Autodesk Inventor part; units mm, degrees
ref_plane "Work Plane1" through (-287.5, 0, 0) normal (0, -1, 0) x (1, 0, 0)
ref_plane "YZ Plane" through (0, 0, 0) normal (1, 0, 0) x (0, 1, 0)
ref_plane "XZ Plane" through (0, 0, 0) normal (0, 1, 0) x (-1, 0, 0)
sketch "Sketch1" plane through (0, 0, 0) normal (0, 0, 1) x (1, 0, 0)
  line L0 (137.5, -75) -> (-137.5, -75)
  line L1 (-137.5, -75) -> (-137.5, 75)
  line L2 (-137.5, 75) -> (137.5, 75)
  line L3 (137.5, 75) -> (137.5, -75)
  line L4 (137.5, -75) -> (-137.5, 75) construction
  line L5 (-137.5, -75) -> (137.5, 75) construction
  line L6 (187.5, 125) -> (-187.5, 125)
  line L7 (-187.5, 125) -> (-187.5, -125)
  line L8 (-187.5, -125) -> (187.5, -125)
  line L9 (187.5, -125) -> (187.5, 125)
  line L10 (-187.5, 125) -> (-287.5, 125)
  line L11 (-287.5, 125) -> (-287.5, 75)
  line L12 (-287.5, 75) -> (-187.5, 75)
  line L13 (-187.5, 75) -> (-187.5, 125)
  line L14 (-187.5, -75) -> (-287.5, -75)
  line L15 (-287.5, -75) -> (-287.5, -125)
  line L16 (-287.5, -125) -> (-187.5, -125)
  line L17 (-187.5, -125) -> (-187.5, -75)
  line L18 (0, 175) -> (0, -175) construction
  line L19 (-1719.5601, 0) -> (1799.9601, 0) construction
  line L20 (187.5, 125) -> (287.5, 125)
  line L21 (287.5, 125) -> (287.5, 75)
  line L22 (287.5, 75) -> (187.5, 75)
  line L23 (187.5, -75) -> (287.5, -75)
  line L24 (287.5, -75) -> (287.5, -125)
  line L25 (287.5, -125) -> (187.5, -125)
  line L26 (1719.5601, 0) -> (-1799.9601, 0) construction
  point P0 (0, 0)
  point P1 (237.5, -125)
  point P2 (0, -125)
  point P3 (-237.5, 125)
  point P4 (0, 125)
  point P5 (237.5, 125)
  point P6 (-237.5, -125)
  point P7 (-237.5, -75)
  point P8 (0, -75)
  point P9 (-237.5, 75)
  point P10 (0, 75)
  point P11 (-287.5, 100)
  point P12 (-287.5, -100)
  point P13 (287.5, 100)
  point P14 (287.5, -100)
  point P15 (187.5, 75)
  dimension "d0" = 50
  dimension "d1" = 150
  dimension "d2" = 275
  dimension "d3" = 100
extrude "Extrusion1" add sketch "Sketch1" along normal blind 30
ref_plane "Work Plane1" through (-287.5, 0, 0) normal (0, -1, 0) x (1, 0, 0)
sketch "Sketch2" plane through (-287.5, 0, 0) normal (0, -1, 0) x (1, 0, 0)
  line L0 (475, 30) -> (475, 0) construction
  line L1 (475, 0) -> (425, 0) construction
  line L2 (425, 0) -> (425, 30) construction
  line L3 (425, 30) -> (475, 30) construction
  line L4 (100, 0) -> (100, 30) construction
  line L5 (100, 30) -> (150, 30) construction
  line L6 (150, 30) -> (150, 0) construction
  line L7 (150, 0) -> (100, 0) construction
  line L8 (475, 30) -> (475, 0) construction
  line L9 (475, 0) -> (425, 0) construction
  line L10 (425, 0) -> (425, 30) construction
  line L11 (100, 0) -> (100, 30) construction
  line L12 (150, 30) -> (150, 0) construction
  line L13 (150, 0) -> (100, 0) construction
  line L14 (0, 0) -> (100, 0) construction
  line L15 (100, 0) -> (100, 30) construction
  line L16 (0, 30) -> (100, 30) construction
  line L17 (0, 0) -> (0, 30) construction
  line L18 (150, 0) -> (425, 0) construction
  line L19 (425, 0) -> (425, 30) construction
  line L20 (150, 30) -> (425, 30) construction
  line L21 (150, 0) -> (150, 30) construction
  line L22 (475, 0) -> (575, 0) construction
  line L23 (575, 0) -> (575, 30) construction
  line L24 (475, 30) -> (575, 30) construction
  line L25 (475, 0) -> (475, 30) construction
  line L26 (0, 0) -> (0, 30)
  line L27 (0, 0) -> (100, 30)
  line L28 (475, 30) -> (575, 0)
  line L29 (425, 30) -> (475, 30)
  line L30 (100, 30) -> (150, 30)
  line L31 (0, 0) -> (100, 0)
  line L32 (100, 30) -> (100, 0)
  line L33 (475, 30) -> (475, 0)
  line L34 (575, 0) -> (0, 0)
  line L35 (575, 0) -> (475, 0)
  line L36 (0, 30) -> (100, 30)
  line L37 (100, 30) -> (100, 0)
  line L38 (100, 0) -> (0, 0)
  line L39 (0, 0) -> (0, 30)
  line L40 (475, 30) -> (575, 30)
  line L41 (575, 30) -> (575, 0)
  line L42 (575, 0) -> (475, 0)
  line L43 (475, 0) -> (475, 30)
  point P0 (287.5, 0)
extrude "Extrusion2" cut sketch "Sketch2" along normal through all both and the other way through all contours L26 L36 L27 | L40 L41 L28
sketch "Sketch3" plane through (-287.5, -125, 0) normal (0, -1, 0) x (1, 0, 0)
  line L0 (475, 0) -> (475, 30)
  line L1 (100, 0) -> (475, 0)
  line L2 (475, 0) -> (475, 15)
  line L3 (475, 15) -> (100, 15)
  line L4 (100, 15) -> (100, 0)
  line L5 (0, 0) -> (575, 0)
  point P0 (287.5, 0)
  point P1 (287.5, 0)
extrude "Extrusion3" cut sketch "Sketch3" against normal through all
ref_plane "Work Plane2" through (-187.5, 0, 30) normal (0, -1, 0) x (1, 0, 0)
ref_plane "Work Plane3" through (0, -75, 30) normal (1, 0, 0) x (0, 0, -1)
properties part number "Base_plartform" material "Stainless Steel"
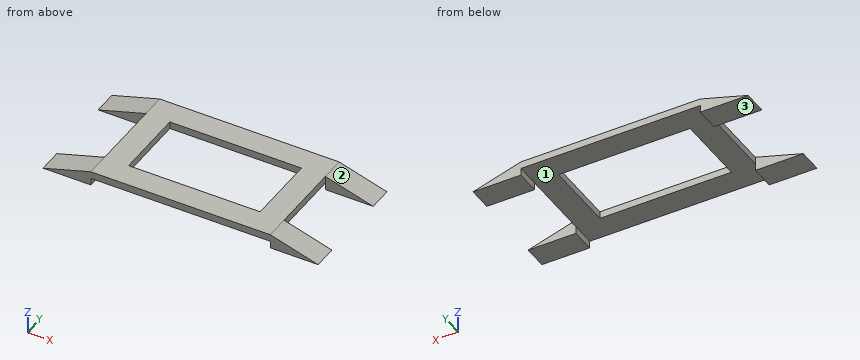
Read the model definition and answer for the solid it produces. Units are mm, in the model's axes. Face numbers are marked on the shaded views. Give positions to 0.01 mm unless a question says otherwise; leave off trailing zeros. Write each loop counter-clockwise with the first axis right and the second up, starting at its lowest first coordinate (ties: lowest second). Pieces come first, ordered by that corner, then holes. Notation, with made-up numbers: (71.5, 27) -> (101.5, 27) arc R17 cw to (101.5, 43) -> close; hole circle Ø10 at (-36.75, -31.75). An arc over 180 degrees is marked (long way). Answer as a JSON object with one key per item and string values. Group by question number.
1) Each of these flat-tipped pins is pushed along its axis until it touches: P1, Ø12, axis at y = 5, z = 21.5, coming from the +X side; P2, Ø2, axis at x = -176.5, y = -35.5, coming from the -Z side; P3, Ø4.5, axis at y = -15.5, z = 26, coming from the -X side; P4, Ø15, axis at x = 252.5, z = 16, coming from the -Y side. Where does it stop, or does it pass through?
2) Consider L1, parallel to Y at x = -18, z = 28; L2, parallel to X at y = -44.5, z = 19.5; L3, parallel to Z at x = 59.5, y = -95. Determine where each line is inside the solid, lowest interval first. Write a range as from..to.
3) The mould has two halves that part along X. Classify the marked faces 1, 2 and 3: +X half, -X half, draft (parallel to the pull), parting line (faces both ways), or undercut.
4) Find section B-B (z = 22.5). Write down the section's boundary in (x, y).
5) Find section C-C (y = 85). Write down the section's boundary in (x, z).
6) Find section A-A (x = -131). Write down the section's boundary in (y, z), and give its area (3 significant figures).
7) Find section D-D (x = -236). Write down the section's boundary in (y, z).
Values follow:
{
 "1": {"P1": "stops at x = 187.5", "P2": "stops at z = 15", "P3": "stops at x = -187.5", "P4": "stops at y = -125"},
 "2": {"L1": "y = -125..-75, 75..125", "L2": "x = -187.5..-137.5, 137.5..187.5", "L3": "z = 15..30"},
 "3": {"face 1": "undercut", "face 2": "+X half", "face 3": "draft"},
 "4": {"outline": "(-212.5, -125) -> (212.5, -125) -> (212.5, -75) -> (187.5, -75) -> (187.5, 75) -> (212.5, 75) -> (212.5, 125) -> (-212.5, 125) -> (-212.5, 75) -> (-187.5, 75) -> (-187.5, -75) -> (-212.5, -75) -> close; hole (-137.5, -75) -> (137.5, -75) -> (137.5, 75) -> (-137.5, 75) -> close"},
 "5": {"outline": "(-287.5, 0) -> (-187.5, 0) -> (-187.5, 15) -> (187.5, 15) -> (187.5, 0) -> (287.5, 0) -> (187.5, 30) -> (-187.5, 30) -> close"},
 "6": {"outline": "(-125, 15) -> (-75, 15) -> (-75, 30) -> (-125, 30) -> close; (75, 15) -> (125, 15) -> (125, 30) -> (75, 30) -> close", "area": "1,500 mm2"},
 "7": {"outline": "(-125, 0) -> (-75, 0) -> (-75, 15.45) -> (-125, 15.45) -> close; (75, 0) -> (125, 0) -> (125, 15.45) -> (75, 15.45) -> close"}
}
